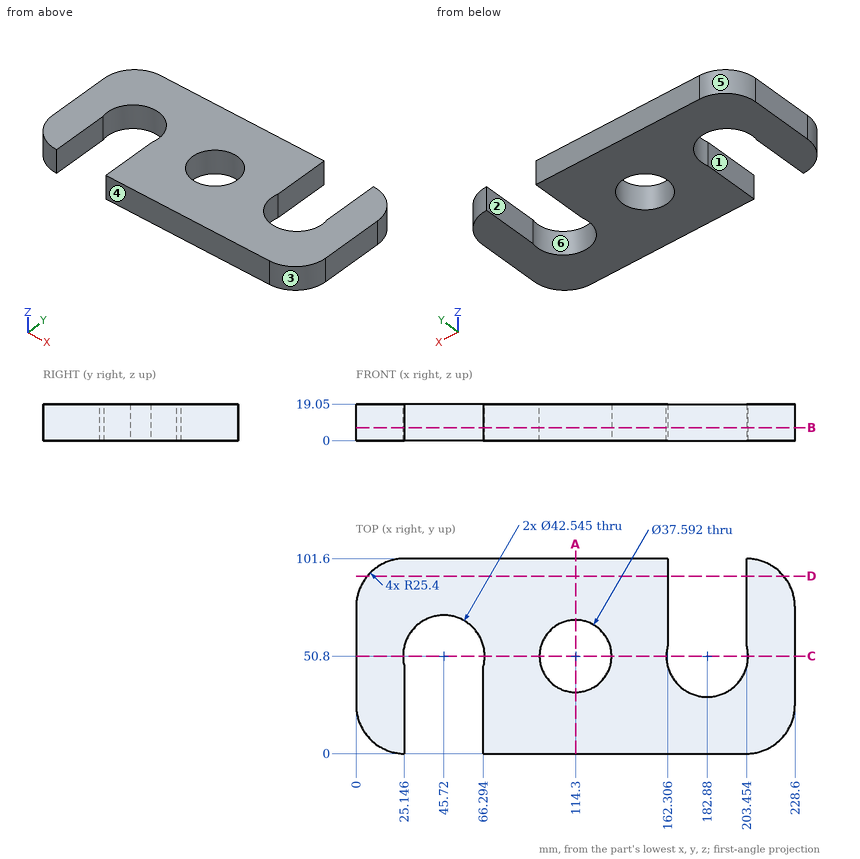
Source: three-view drawing plus pictorial views. Frame: mm from the lowest corner of the part. A direction names the side the tool comes from. Round coordinates to 2 decimals unless told otherwise and drop trailing zeros. Write each loop counter-clockwise with the first axis right and the second up, starting at its lowest first coordinate (ties: lowest second). Pieces come first, ordered by that corner, then holes. Notation, with made-up numbers: M -15,15.25 L 37,15.25 A21 cw 37,54.25 Z; hole C 22,50 d1. An arc over 180 degrees is marked long. Write item = value, one per line.
Item 1: Section query D-D on y = 92.5. Return loops of the section in (x, z), then the cut area to 3 significant figures.
Findings:
outline = M 5.92,0 L 162.31,0 L 162.31,19.05 L 5.92,19.05 Z; M 203.45,0 L 222.68,0 L 222.68,19.05 L 203.45,19.05 Z
area = 3,350 mm^2
Item 2: Pin query (flat end, axial travel): P1, Ø9.5, axis at y = 18.5, z = 7, coming from the +X side; P2, Ø3, axis at y = 18, z = 3.5, coming from the -X side; P3, Ø5.5, axis at y = 90, z = 13, coming from the +X side. Return the tip coordinate at first contact, or that it passes through.
Findings:
P1 = 228.51
P2 = 0.69
P3 = 226.07
Item 3: Pull-direction query (Y, two-part tool) for the marked faces 4, 5 and 6; classes: pulls with the +Y half, pulls with the -Y half, needs draft (parallel to the pull), parting line crosses it, or undercut.
Findings:
face_4 = pulls with the -Y half
face_5 = pulls with the +Y half
face_6 = undercut
Item 4: Section query A-A on x = 114.3. Return loops of the section in (y, z).
Findings:
outline = M 0,0 L 32,0 L 32,19.05 L 0,19.05 Z; M 69.6,0 L 101.6,0 L 101.6,19.05 L 69.6,19.05 Z
Item 5: Section query C-C on y = 50.8. Return loops of the section in (x, z), then the cut area to 3 significant figures.
Findings:
outline = M 0,0 L 24.45,0 L 24.45,19.05 L 0,19.05 Z; M 66.99,0 L 95.5,0 L 95.5,19.05 L 66.99,19.05 Z; M 133.1,0 L 161.61,0 L 161.61,19.05 L 133.1,19.05 Z; M 204.15,0 L 228.6,0 L 228.6,19.05 L 204.15,19.05 Z
area = 2,020 mm^2
Item 6: Section query B-B on z = 6.75. Return loops of the section in (x, y) (1 decimal).
Findings:
outline = M 0,25.4 A25.4 ccw 25.1,0 L 25.1,45.4 A21.3 cw long 66.3,45.4 L 66.3,0 L 203.2,0 A25.4 ccw 228.6,25.4 L 228.6,76.2 A25.4 ccw 203.5,101.6 L 203.5,56.2 A21.3 cw long 162.3,56.2 L 162.3,101.6 L 25.4,101.6 A25.4 ccw 0,76.2 Z; hole C 114.3,50.8 d37.6
Item 7: Access query for the marked faces 1, 2 and 3. Directions: +Z, -Z, +X, -X, +Y, -Y. A direction counts if a zero-diameter tool reaches every point of the face in a straight line with its end or side. Return the directions, or none.
Findings:
face_1 = +Z, -Z, -Y
face_2 = +Z, -Z, +Y
face_3 = +Z, -Z, +X, -Y
Item 8: Material intervals for line 1 along X through (y, z) = (75.5, 13.5); line 2 along X through (y, z) = (38, 9.25); line 3 along X through (y, z) = (16.5, 4.5), sorted ascending. Write a range as [from, to].
Findings:
line_1 = [0, 162.31], [203.45, 228.6]
line_2 = [0, 25.15], [66.29, 100.54], [128.06, 165.89], [199.87, 228.6]
line_3 = [1.61, 25.15], [66.29, 226.99]
